Check sheet for the modelled part. Datum: model origin and axes. Units: mm. A direction names the side the tool comes from. Give positions to 0.01 mm unless a question says otherwise; leave off trailing zeros. Order: outer loops, then holes, each group sorted by start corner. A loop starts at its lowest first (then second) coordinate and runs counter-clockwise, first axis right, second up. Notation, with made-up numbers: M 6.25,1 L 59.25,1 A16 ccw 59.25,29 Z; hole C 88,67.25 d8. An arc over 180 degrees is marked long. One line per question, with ' | ' between items. Start each with the question number.
```python
from build123d import *

# Parameters (mm, degrees)
BOSS_EXTRUDE1_DEPTH = 4
SKETCH2_R           = 1.5875
CUT_EXTRUDE1_DEPTH  = 10
FILLET1_R           = 1
SKETCH3_W           = 4.5
SKETCH3_H           = 0.2
CUT_EXTRUDE2_DEPTH  = 10
FILLET2_R           = 1
SKETCH4_R           = 1.190625
CUT_EXTRUDE3_DEPTH  = 10


with BuildPart() as part:
    # Sketch1 → Boss-Extrude1 (new body, symmetric)
    with BuildSketch(Plane.XY):
        Polygon((0, 0), (6, 0), (9, 3.625), (21, 3.625), (21, 3.825), (8.905909928, 3.825), (5.905909928, 0.2), (0, 0.2), align=None)
    extrude(amount=BOSS_EXTRUDE1_DEPTH, both=True)

    # Sketch2 → Cut-Extrude1 (cut)
    with BuildSketch(Plane(origin=(0, 3.825, 0), x_dir=(1, 0, 0), z_dir=(0, 1, 0))):
        with Locations((17.705909928, 0)):
            Circle(SKETCH2_R)
    extrude(amount=-CUT_EXTRUDE1_DEPTH, mode=Mode.SUBTRACT)

    # Fillet1
    fillet1_edges = [part.edges().sort_by_distance(p)[0] for p in [
        (0, 0.1, -4),
        (21, 3.725, 4),
        (0, 0.1, 4),
        (21, 3.725, -4),
    ]]
    fillet(fillet1_edges, radius=FILLET1_R)

    # Sketch3 → Cut-Extrude2 (cut)
    with BuildSketch(Plane(origin=(0, 0.2, 0), x_dir=(1, 0, 0), z_dir=(0, 1, 0))):
        with Locations((2.25, 0)):
            Rectangle(SKETCH3_W, SKETCH3_H)
    extrude(amount=-CUT_EXTRUDE2_DEPTH, mode=Mode.SUBTRACT)

    # Fillet2
    fillet2_edges = [part.edges().sort_by_distance(p)[0] for p in [
        (5.905909928, 0.2, 0),
        (8.905909928, 3.825, 0),
    ]]
    fillet(fillet2_edges, radius=FILLET2_R)

    # Sketch4 → Cut-Extrude3 (cut)
    with BuildSketch(Plane(origin=(3.406965596, -2.819557735, 0), x_dir=(0, 0, 1), z_dir=(-0.770394321, 0.637567714, 0))):
        with Locations((-1.75, 6.272187634)):
            Circle(SKETCH4_R)
    cut_extrude3 = extrude(amount=-CUT_EXTRUDE3_DEPTH, mode=Mode.SUBTRACT)

    # Mirror1: Cut-Extrude3 across plane
    add(cut_extrude3.mirror(Plane.XY), mode=Mode.SUBTRACT)


solid = part.part
```
Item 1: Section check C-C, the plane z = -2.5. Record the cut outline in (x, y) (3 decimals).
Item 2: Section check B-B, the plane z = 0.75. Record the cut outline in (x, y) (3 decimals).
Item 3: Section check A-A, the plane x = 4. Record the cut outline in (y, z), then the cut area to 3 significant figures.
Item 4: Set-up check for faces 1 (the face through (15, 3.625, 0)), 2 (the face through (15, 3.825, 0)), 3 (the face through (3, 0.2, 1)): record each of +Z, -Z, +X, -X, +Y, -Y from which the full face is reachable in a straight line by a thin tool's end or side.
Item 5: Scan lines: probe 1 along Y at (x, z) = (10.5, 0.5) (3 decimals); probe 2 along Y at (x, z) = (4.75, 3); probe 3 along X at (y, z) = (3.7, 0). Record each from-to range of solid material in increasing order. Write a range as [from, to].
Item 6: Go/stop test with flat-tipped pins: P1, Ø1, axis at x = 7, z = 0, coming from the +Y side; P2, Ø4, axis at x = 12.5, z = -2, coming from the -Y side (3 decimals); P3, Ø3, axis at x = 17.71, z = 0, coming from the +Y side; P4, Ø4, axis at x = 3.5, z = -1, coming from the +Y side. Record where each tip stops, or that it passes through.
Reported:
1) outline: M 0,0 L 6,0 L 6.97,1.173 L 6.816,1.3 L 6.206,0.562 A1 cw 5.435,0.2 L 0,0.2 Z; M 7.995,2.725 L 8.15,2.597 L 9,3.625 L 21,3.625 L 21,3.825 L 9.376,3.825 A1 ccw 8.606,3.463 Z
2) outline: M 0,0 L 6,0 L 7.148,1.387 L 6.994,1.515 L 6.206,0.562 A1 cw 5.435,0.2 L 0,0.2 Z; M 7.818,2.51 L 7.972,2.383 L 9,3.625 L 16.307,3.625 L 16.307,3.825 L 9.376,3.825 A1 ccw 8.606,3.463 Z; M 19.105,3.625 L 21,3.625 L 21,3.825 L 19.105,3.825 Z
3) outline: M 0,-4 L 0.2,-4 L 0.2,-0.1 L 0,-0.1 Z; M 0,0.1 L 0.2,0.1 L 0.2,4 L 0,4 Z | area: 1.56 mm^2
4) face 1: +Z, -Z, +X, -Y | face 2: +Z, -Z, +X, -X, +Y | face 3: +Z, -Z, -X, +Y
5) probe 1: y = [3.625, 3.825] | probe 2: y = [0, 0.2] | probe 3: x = [8.89, 16.12], [19.29, 21]
6) P1: stops at y = 2.13 | P2: stops at y = 3.625 | P3: passes through | P4: stops at y = 0.2
